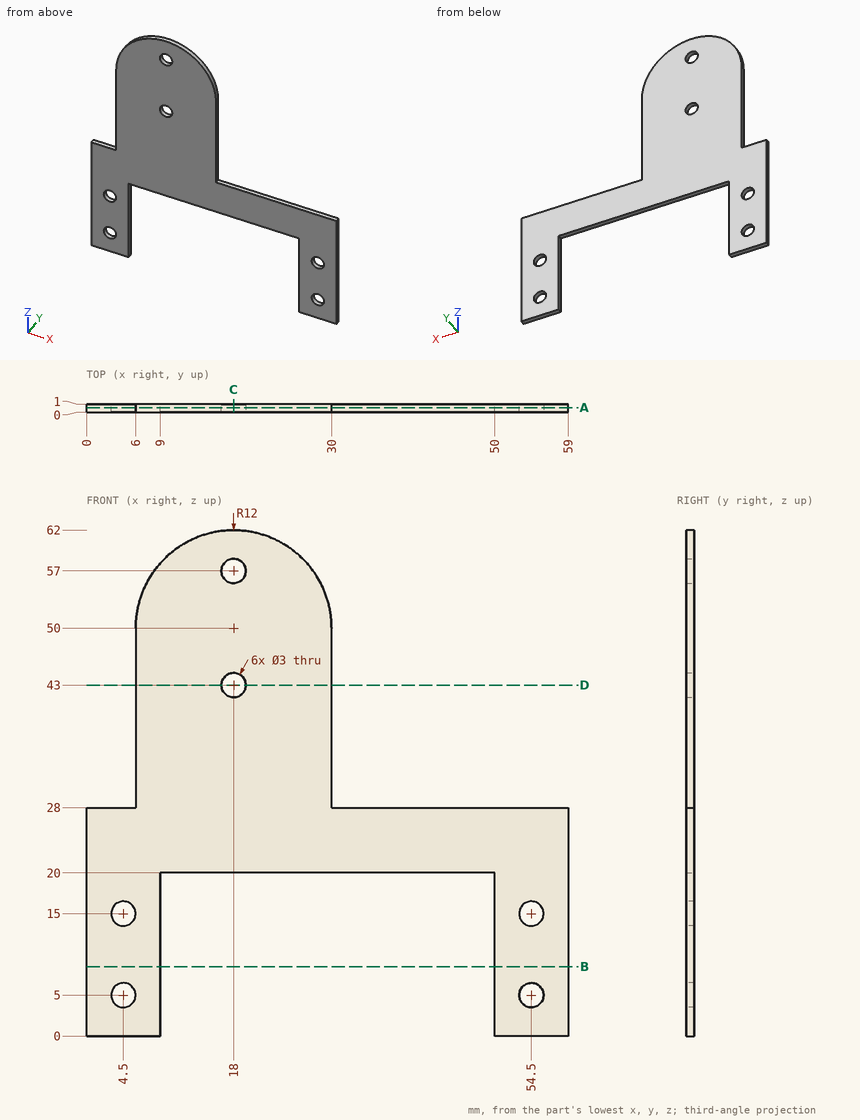
Study the drawing (mm; zero at the part's minimum x, y, z) and answer. Give positions to 0.01 mm unless a question says otherwise; leave off trailing zeros. Write each loop counter-clockwise with the first axis right and the second up, starting at its lowest first coordinate (ties: lowest second). Pieces come first, ordered by that corner, then holes. Notation, with made-up numbers: (34.5, 8) - (71.5, 8) arc R25 ccw to (71.5, 47) - close; hole circle Ø2 at (70, 77.25). An arc over 180 degrees is marked (long way). Write item = value, one per line. Start each with the question number.
Item 1: Find section D-D (z = 43). Give the vertices of the cut face in (x, y), then the cut area to 3 significant figures.
Item 2: Each of these flat-tipped pins is pushed along its axis until it touches: P1, Ø4, axis at x = 4.5, z = 15, coming from the -Y side; P2, Ø0.5, axis at x = 45.5, y = 0.5, coming from the +Z side. Where does it stop, or does it pass through?
Item 3: Find section B-B (z = 8.5). Give the vertices of the cut face in (x, y).
Item 4: Find section A-A (y = 0.55). Give the vertices of the cut face in (x, z).
Item 5: Find the intervals of material crossed by probe 1 along Z at (x, y) = (18, 0.5); probe 2 along X at (y, z) = (0.5, 15); probe 3 along Z at (x, y) = (4.5, 0.7), in increasing order. Write a range as [from, to].
Item 6: Find section C-C (x = 18). Give the vertices of the cut face in (y, z), then the cut area to 3 significant figures.
Response:
q1.outline = (6, 0) - (16.5, 0) - (16.5, 1) - (6, 1) - close; (19.5, 0) - (30, 0) - (30, 1) - (19.5, 1) - close
q1.area = 21.0 mm²
q2.P1 = 0
q2.P2 = 28
q3.outline = (0, 0) - (9, 0) - (9, 1) - (0, 1) - close; (50, 0) - (59, 0) - (59, 1) - (50, 1) - close
q4.outline = (0, 0) - (9, 0) - (9, 20) - (50, 20) - (50, 0) - (59, 0) - (59, 28) - (30, 28) - (30, 50) arc R12 ccw to (6, 50) - (6, 28) - (0, 28) - close; hole circle Ø3 at (4.5, 5); hole circle Ø3 at (4.5, 15); hole circle Ø3 at (18, 43); hole circle Ø3 at (18, 57); hole circle Ø3 at (54.5, 5); hole circle Ø3 at (54.5, 15)
q5.probe_1 = [20, 41.5], [44.5, 55.5], [58.5, 62]
q5.probe_2 = [0, 3], [6, 9], [50, 53], [56, 59]
q5.probe_3 = [0, 3.5], [6.5, 13.5], [16.5, 28]
q6.outline = (0, 20) - (1, 20) - (1, 41.5) - (0, 41.5) - close; (0, 44.5) - (1, 44.5) - (1, 55.5) - (0, 55.5) - close; (0, 58.5) - (1, 58.5) - (1, 62) - (0, 62) - close
q6.area = 36.0 mm²
